from build123d import *

# Parameters (mm, degrees)
EXTRUDE_1_DEPTH     = 6
SKETCH_2_R          = 18.75
CUT_EXTRUDE_1_DEPTH = 1


with BuildPart() as part:
    # 草图1 → 凸台-拉伸1 (new body)
    with BuildSketch(Plane.XY):
        with BuildLine():
            Line((0, 30), (40, 30))
            Line((40, 30), (40, -30))
            Line((40, -30), (0, -30))
            ThreePointArc((0, -30), (-30, 0), (0, 30))
        make_face()
    extrude(amount=EXTRUDE_1_DEPTH)

    # 草图2 → 切除-拉伸1 (cut)
    with BuildSketch(Plane(origin=(0, 0, 0), x_dir=(-1, 0, 0), z_dir=(0, 0, -1))):
        Circle(SKETCH_2_R)
    extrude(amount=-CUT_EXTRUDE_1_DEPTH, mode=Mode.SUBTRACT)


solid = part.part
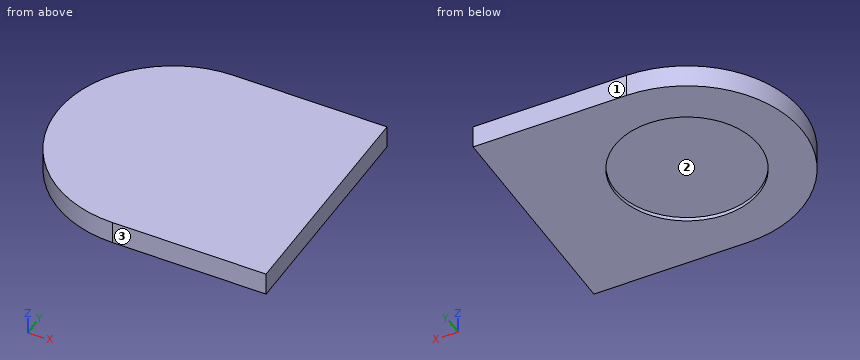
Geometry: final body of the model. Coordinates: model frame, mm. Face numbers are marked on the shaded views. Give positions to 0.01 mm unless a question says otherwise; leave off trailing zeros. Order: outer loops, then holes, each group sorted by start corner. A loop starts at its lowest first (then second) coordinate and runs counter-clockwise, first axis right, second up. Notation, with made-up numbers: (53.5, 72) -> (89.5, 72) arc R6 ccw to (89.5, 83) -> close; hole circle Ø9 at (-9.5, 42.5). An arc over 180 degrees is marked (long way). Write each question's results on one line, items separated by ' | '.
1) Line query: line 1 along Y through (x, z) = (0, 0.5); line 2 along Z through (x, y) = (-0.5, -8); line 3 along X through (y, z) = (-3, 1.7). Output: solid intervals per line, ascending.
Geometry says:
line 1: y = -30 to -18.75, 18.75 to 30 | line 2: z = 1 to 6 | line 3: x = -29.85 to 40
2) Cut plane B-B (x = -17). Output: boundary loops of the cut face in (y, z), and give its area (3 significant figures).
Geometry says:
outline: (-24.72, 0) -> (-7.91, 0) -> (-7.91, 1) -> (7.91, 1) -> (7.91, 0) -> (24.72, 0) -> (24.72, 6) -> (-24.72, 6) -> close | area: 281 mm²
3) Draft query along Y for the marked faces 1, 2 and 3. Return one class per face: released by +Y, released by -Y, zero draft, split by the parting line, or undercut.
Geometry says:
face 1: released by +Y | face 2: undercut | face 3: released by -Y
4) Cut plane A-A (y = 0). Output: boundary loops of the cut face in (x, z).
Geometry says:
outline: (-30, 0) -> (-18.75, 0) -> (-18.75, 1) -> (18.75, 1) -> (18.75, 0) -> (40, 0) -> (40, 6) -> (-30, 6) -> close
5) First-contact query: pin 1 Ø1 at (y, z) = (9, 2.5) entering from -X; pin 2 Ø11 at (x, y) = (-1, 6) entering from -Z. Flat tips, straight axial feed; report the tip coordinate or a pass-through.
Geometry says:
pin 1: stops at x = -28.77 | pin 2: stops at z = 1
6) Cut plane C-C (z = 4.55). Output: boundary loops of the cut face in (x, y), and give its area (3 significant figures).
Geometry says:
outline: (0, -30) -> (40, -30) -> (40, 30) -> (0, 30) arc R30 ccw to start | area: 3,810 mm²
